Build history of the part. All positions in model axes, mm. Coordinates: 2 decimals unless noted, no trailing zeros. Loops run counter-clockwise (first coordinate to the right, second up) from the corner with the lowest first, then second, coordinate; pieces in that order, holes last.
Item 1: Cut at A-A (x = 16.5). List the corners of the cut face in (y, z), and give its area (3 significant figures).
Item 2: Drill centre lines: line 1 along X through (y, z) = (387, 4.45); line 2 along Y through (x, z) = (0, 1.9); line 3 along Y through (x, z) = (-48.5, 2.85). Where is each one in solid material? Low to high.
Item 3: Cut at C-C (z = 3.5). List the corners of the cut face in (x, y).
Item 4: Cut at B-B (y = 369.5). List the corners of the cut face in (x, z), and give its area (3 significant figures).
from build123d import *

# Parameters (mm, degrees)
SKETCH_1_W          = 279.576527547
SKETCH_1_H          = 4
EXTRUDE_1_DEPTH     = 533.213673317
SKETCH_2_R          = 20
CUT_EXTRUDE_1_DEPTH = 553.536377523
SKETCH1_W           = 155
SKETCH1_H           = 320
CUT_EXTRUDE1_DEPTH  = 553.536377523


with BuildPart() as part:
    # Эскиз1 → Вытянуть1 (new body)
    with BuildSketch(Plane(origin=(0, 0, 0), x_dir=(1, 0, 0), z_dir=(0, 1, 0))):
        with Locations((-4.999950783, -3.341392103)):
            Rectangle(SKETCH_1_W, SKETCH_1_H)
    extrude(amount=EXTRUDE_1_DEPTH)

    # Эскиз2 → Вырез-Вытянуть1 (cut, through all)
    with BuildSketch(Plane(origin=(0, 0, 1.341392103), x_dir=(-1, 0, 0), z_dir=(0, 0, -1))):
        with Locations((64.651566286, 68.554150891)):
            Circle(SKETCH_2_R)
    extrude(amount=-CUT_EXTRUDE_1_DEPTH, mode=Mode.SUBTRACT)

    # Sketch1 → Cut-Extrude1 (cut, through all)
    with BuildSketch(Plane(origin=(0, 0, 1.341392103), x_dir=(-1, 0, 0), z_dir=(0, 0, -1))):
        with Locations((4.999950782, 288.213673317)):
            Rectangle(SKETCH1_W, SKETCH1_H)
    extrude(amount=-CUT_EXTRUDE1_DEPTH, mode=Mode.SUBTRACT)


solid = part.part
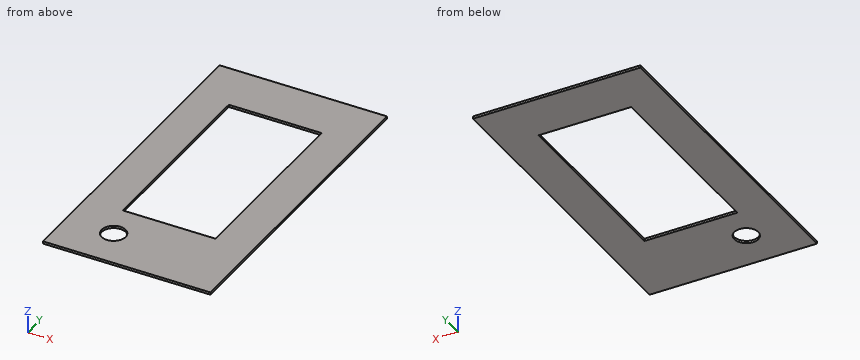
Filled sheet:
1. outline: (0, 1.34) - (128.21, 1.34) - (128.21, 5.34) - (0, 5.34) - close; (448.21, 1.34) - (533.21, 1.34) - (533.21, 5.34) - (448.21, 5.34) - close
1. area: 853 mm2
2. line 1: x = -144.79 to -82.5, 72.5 to 134.79
2. line 2: y = 0 to 128.21, 448.21 to 533.21
2. line 3: y = 0 to 56.76, 80.35 to 128.21, 448.21 to 533.21
3. outline: (-144.79, 0) - (134.79, 0) - (134.79, 533.21) - (-144.79, 533.21) - close; hole circle Ø40 at (-64.65, 68.55); hole (-82.5, 128.21) - (72.5, 128.21) - (72.5, 448.21) - (-82.5, 448.21) - close
4. outline: (-144.79, 1.34) - (-82.5, 1.34) - (-82.5, 5.34) - (-144.79, 5.34) - close; (72.5, 1.34) - (134.79, 1.34) - (134.79, 5.34) - (72.5, 5.34) - close
4. area: 498 mm2
